Build history of the part. All positions in model axes, mm. Face numbers are marked on the shaded views. Round coordinates to 2 decimals unless told otherwise and drop trailing zeros. Write each loop counter-clockwise with the first axis right and the second up, starting at its lowest first coordinate (ties: lowest second). Pieces come first, ordered by that corner, then holes.
1) Flat gauge pin, fed straight in: pin 1 (1 mm diameter, centred on x = 14.5, y = 4, fed in from +Z). Where does the tip first touch, or does it go through?
2) Pull direction Y, two halves, no side cores. Call the marked faces 1, 2, 3 and 4: +Y half, -Y half, draft (parallel to the pull), parting line (faces both ways), or undercut.
3) Saw through at A-A (z = 42). Write the cut outline in (x, y), plus the area to 3 significant figures.
4) Saw through at C-C (z = 26). Write the cut outline in (x, y).
5) Wall check: probe 1 along Y at (x, z) = (11, 6); probe 2 along Z at (x, y) = (11, 26); probe 3 along X at (y, z) = (36.5, 27.5). Give the ranges that are in metal, low to high.
6) Saw through at B-B (y = -6). Write the cut outline in (x, z).
from build123d import *

# Parameters (mm, degrees)
EXTRUDE_1_DEPTH     = 3
SKETCH_2_W          = 32
SKETCH_2_H          = 3
EXTRUDE_2_DEPTH     = 56
SKETCH_3_R          = 1.65
SKETCH_3_R_2        = 12
SKETCH_3_W          = 20
SKETCH_3_H          = 40
CUT_EXTRUDE_2_DEPTH = 58
FILLET_1_R          = 2


with BuildPart() as part:
    # 草图1 → 凸台-拉伸1 (new body)
    with BuildSketch(Plane.XY):
        with BuildLine():
            Line((0, 12), (0, 0))
            Line((0, 0), (0, -15))
            Line((0, -15), (16, -15))
            Line((16, -15), (16, 2.35))
            ThreePointArc((16, 2.35), (14.833273811, 2.833273811), (14.35, 4))
            Line((14.35, 4), (9.65, 4))
            ThreePointArc((9.65, 4), (6.833273811, 2.833273811), (8, 5.65))
            Line((8, 5.65), (8, 10.35))
            ThreePointArc((8, 10.35), (6.35, 12), (8, 13.65))
            Line((8, 13.65), (8, 18.35))
            ThreePointArc((8, 18.35), (6.833273811, 21.166726189), (9.65, 20))
            Line((9.65, 20), (14.35, 20))
            ThreePointArc((14.35, 20), (14.833273811, 21.166726189), (16, 21.65))
            Line((16, 21.65), (16, 39))
            Line((16, 39), (0, 39))
            Line((0, 39), (0, 24))
            Line((0, 24), (0, 12))
        make_face()
        with BuildLine():
            Line((32, 39), (16, 39))
            Line((16, 39), (16, 21.65))
            ThreePointArc((16, 21.65), (17.166726189, 21.166726189), (17.65, 20))
            Line((17.65, 20), (22.35, 20))
            ThreePointArc((22.35, 20), (24, 21.65), (25.65, 20))
            ThreePointArc((25.65, 20), (25.166726189, 18.833273811), (24, 18.35))
            Line((24, 18.35), (24, 13.65))
            ThreePointArc((24, 13.65), (25.166726189, 13.166726189), (25.65, 12))
            Line((25.65, 12), (32, 12))
            Line((32, 12), (32, 24))
            Line((32, 24), (32, 39))
        make_face()
        with BuildLine():
            Line((16, 2.35), (16, -15))
            Line((16, -15), (32, -15))
            Line((32, -15), (32, 0))
            Line((32, 0), (32, 12))
            Line((32, 12), (25.65, 12))
            ThreePointArc((25.65, 12), (25.166726189, 10.833273811), (24, 10.35))
            Line((24, 10.35), (24, 5.65))
            ThreePointArc((24, 5.65), (25.166726189, 5.166726189), (25.65, 4))
            ThreePointArc((25.65, 4), (24, 2.35), (22.35, 4))
            Line((22.35, 4), (17.65, 4))
            ThreePointArc((17.65, 4), (17.166726189, 2.833273811), (16, 2.35))
        make_face()
        with BuildLine():
            ThreePointArc((16, 18.35), (14.833273811, 18.833273811), (14.35, 20))
            Line((14.35, 20), (9.65, 20))
            ThreePointArc((9.65, 20), (9.166726189, 18.833273811), (8, 18.35))
            Line((8, 18.35), (8, 13.65))
            ThreePointArc((8, 13.65), (9.166726189, 13.166726189), (9.65, 12))
            Line((9.65, 12), (14.35, 12))
            ThreePointArc((14.35, 12), (14.833273811, 13.166726189), (16, 13.65))
            Line((16, 13.65), (16, 18.35))
        make_face()
        with BuildLine():
            Line((22.35, 20), (17.65, 20))
            ThreePointArc((17.65, 20), (17.166726189, 18.833273811), (16, 18.35))
            Line((16, 18.35), (16, 13.65))
            ThreePointArc((16, 13.65), (17.166726189, 13.166726189), (17.65, 12))
            Line((17.65, 12), (22.35, 12))
            ThreePointArc((22.35, 12), (22.833273811, 13.166726189), (24, 13.65))
            Line((24, 13.65), (24, 18.35))
            ThreePointArc((24, 18.35), (22.833273811, 18.833273811), (22.35, 20))
        make_face()
        with BuildLine():
            Line((9.65, 4), (14.35, 4))
            ThreePointArc((14.35, 4), (14.833273811, 5.166726189), (16, 5.65))
            Line((16, 5.65), (16, 10.35))
            ThreePointArc((16, 10.35), (14.833273811, 10.833273811), (14.35, 12))
            Line((14.35, 12), (9.65, 12))
            ThreePointArc((9.65, 12), (9.166726189, 10.833273811), (8, 10.35))
            Line((8, 10.35), (8, 5.65))
            ThreePointArc((8, 5.65), (9.166726189, 5.166726189), (9.65, 4))
        make_face()
        with BuildLine():
            ThreePointArc((16, 5.65), (17.166726189, 5.166726189), (17.65, 4))
            Line((17.65, 4), (22.35, 4))
            ThreePointArc((22.35, 4), (22.833273811, 5.166726189), (24, 5.65))
            Line((24, 5.65), (24, 10.35))
            ThreePointArc((24, 10.35), (22.833273811, 10.833273811), (22.35, 12))
            Line((22.35, 12), (17.65, 12))
            ThreePointArc((17.65, 12), (17.166726189, 10.833273811), (16, 10.35))
            Line((16, 10.35), (16, 5.65))
        make_face()
    extrude(amount=EXTRUDE_1_DEPTH)

    # 草图2 → 凸台-拉伸2 (add)
    with BuildSketch(Plane.XY.offset(3)):
        with Locations((16, 37.5)):
            Rectangle(SKETCH_2_W, SKETCH_2_H)
        with Locations((16, -13.5)):
            Rectangle(SKETCH_2_W, SKETCH_2_H)
    extrude(amount=EXTRUDE_2_DEPTH)

    # 草图3 → 切除-拉伸2 (cut)
    with BuildSketch(Plane(origin=(0, 39, 0), x_dir=(1, 0, 0), z_dir=(0, 1, 0))):
        with Locations((6, -52)):
            Circle(SKETCH_3_R)
        with Locations((6, -32)):
            Circle(SKETCH_3_R)
        with Locations((6, -12)):
            Circle(SKETCH_3_R)
        with Locations((26, -12)):
            Circle(SKETCH_3_R)
        with Locations((26, -52)):
            Circle(SKETCH_3_R)
        with Locations((26, -32)):
            Circle(SKETCH_3_R)
        with Locations((16, -42)):
            Circle(SKETCH_3_R_2)
        with Locations((16, -22)):
            Circle(SKETCH_3_R_2)
        with Locations((16, -32)):
            Rectangle(SKETCH_3_W, SKETCH_3_H)
    extrude(amount=-CUT_EXTRUDE_2_DEPTH, mode=Mode.SUBTRACT)

    # 圆角1
    fillet_1_edges = [part.edges().sort_by_distance(p)[0] for p in [
        (0, 37.5, 59),
        (32, 37.5, 59),
        (32, -13.5, 59),
        (0, -13.5, 59),
    ]]
    fillet(fillet_1_edges, radius=FILLET_1_R)


solid = part.part
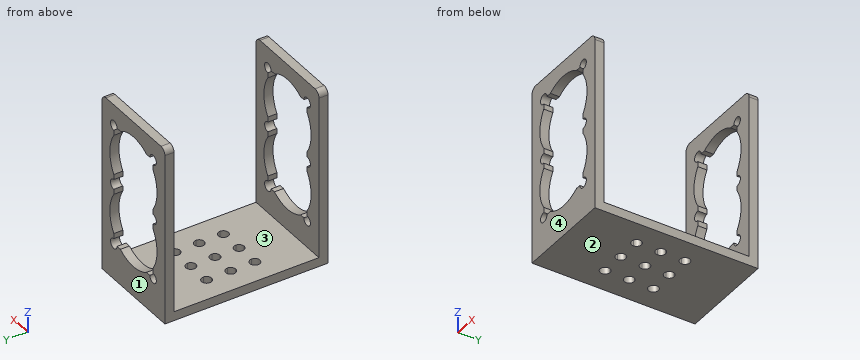
Evaluation:
1. pin 1: stops at z = 3
2. face 1: +Y half
2. face 2: draft
2. face 3: undercut
2. face 4: -Y half
3. outline: (0, -15) - (4, -15) - (4, -12) - (0, -12) - close; (0, 36) - (4, 36) - (4, 39) - (0, 39) - close; (28, -15) - (32, -15) - (32, -12) - (28, -12) - close; (28, 36) - (32, 36) - (32, 39) - (28, 39) - close
3. area: 48.0 mm2
4. outline: (0, -15) - (4.69, -15) - (4.69, -12) - (0, -12) - close; (0, 36) - (4.69, 36) - (4.69, 39) - (0, 39) - close; (27.31, -15) - (32, -15) - (32, -12) - (27.31, -12) - close; (27.31, 36) - (32, 36) - (32, 39) - (27.31, 39) - close
5. probe 1: y = -15 to -12, 36 to 39
5. probe 2: z = 0 to 3
5. probe 3: x = 0 to 5.33, 26.67 to 32
6. outline: (0, 0) - (32, 0) - (32, 3) - (0, 3) - close
